Can you work these out from the drawing? Everything is in mm from the part's minimum corner. Give positions to 0.01 mm unless a question says otherwise; leave off trailing zeros. Write each loop counter-clockwise with the first axis right and the second up, starting at its lowest first coordinate (ties: lowest second). Pieces come first, ordered by that corner, then holes. Notation, with made-up numbers: (74, -20.5) - (97, -20.5) arc R29 cw to (97, 4.5) - close; hole circle Ø4 at (-2, 43.5). An arc over 180 degrees is marked (long way). Use a Markdown table: item, result.
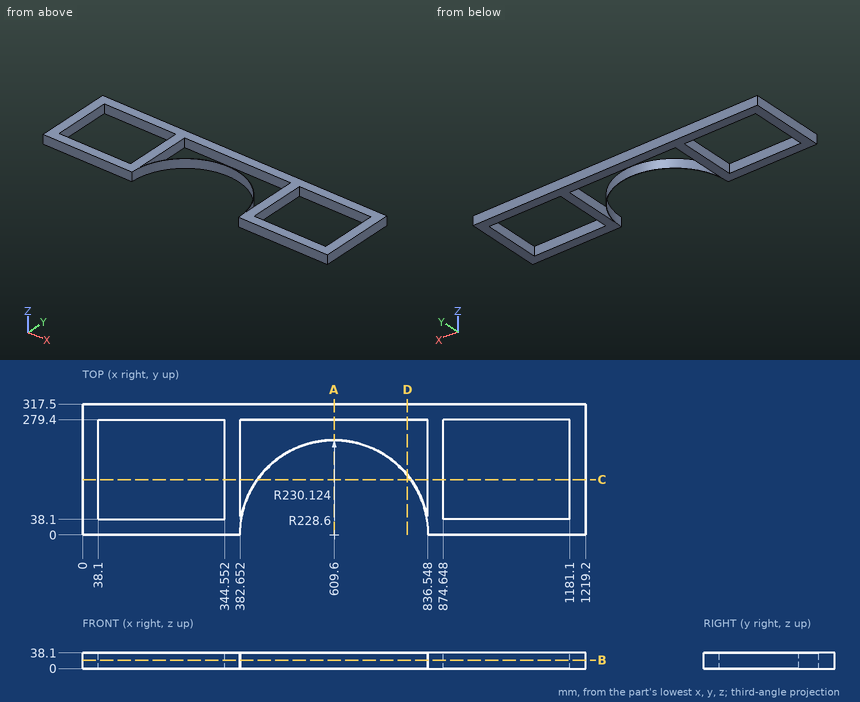
Item 1: If we section it at D-D, the plane x = 787.5: Write out the boundary of the cut face in (y, z) (3 decimals), plus the area to 3 significant figures.
Values:
| item | result |
|---|---|
| outline | (143.56, 0) - (145.975, 0) - (145.975, 38.1) - (143.56, 38.1) - close; (279.4, 0) - (317.5, 0) - (317.5, 38.1) - (279.4, 38.1) - close |
| area | 1,540 mm2 |
Item 2: If we section it at C-C, the plane y = 134: Write out the boundary of the cut face in (x, z).
Values:
| item | result |
|---|---|
| outline | (0, 0) - (38.1, 0) - (38.1, 38.1) - (0, 38.1) - close; (344.55, 0) - (382.65, 0) - (382.65, 38.1) - (344.55, 38.1) - close; (422.51, 0) - (424.39, 0) - (424.39, 38.1) - (422.51, 38.1) - close; (794.81, 0) - (796.69, 0) - (796.69, 38.1) - (794.81, 38.1) - close; (836.55, 0) - (874.65, 0) - (874.65, 38.1) - (836.55, 38.1) - close; (1181.1, 0) - (1219.2, 0) - (1219.2, 38.1) - (1181.1, 38.1) - close |
Item 3: If we section it at A-A, the plane x = 609.6: Write out the boundary of the cut face in (y, z).
Values:
| item | result |
|---|---|
| outline | (228.6, 0) - (230.12, 0) - (230.12, 38.1) - (228.6, 38.1) - close; (279.4, 0) - (317.5, 0) - (317.5, 38.1) - (279.4, 38.1) - close |
Item 4: Will this pin go through, and if not, where does the flat tip stop? pin 1 Ø19 at (x, z) = (533, 15) entering from -Y.
Values:
| item | result |
|---|---|
| pin 1 | stops at y = 211.77 |
Item 5: I need wall thicknesses on line 1 along Y through (x, z) = (118, 15.5); line 2 along X through (y, z) = (210, 11); line 3 along X through (y, z) = (160, 26). Which ranges of each line are inside material? Lowest first, please. Write a range as [from, to].
Values:
| item | result |
|---|---|
| line 1 | y = [0, 38.1], [279.4, 317.5] |
| line 2 | x = [0, 38.1], [344.55, 382.65], [515.49, 519.28], [699.92, 703.71], [836.55, 874.65], [1181.1, 1219.2] |
| line 3 | x = [0, 38.1], [344.55, 382.65], [444.2, 446.33], [772.87, 775], [836.55, 874.65], [1181.1, 1219.2] |
Item 6: If we section it at B-B, the plane z = 21: Write out the boundary of the cut face in (x, y).
Values:
| item | result |
|---|---|
| outline | (0, 0) - (381, 0) arc R228.6 cw to (838.2, 0) - (1219.2, 0) - (1219.2, 317.5) - (0, 317.5) - close; hole (38.1, 38.1) - (344.55, 38.1) - (344.55, 279.4) - (38.1, 279.4) - close; hole (382.65, 38.1) arc R230.12 cw to (836.55, 38.1) - (836.55, 279.4) - (382.65, 279.4) - close; hole (874.65, 38.1) - (1181.1, 38.1) - (1181.1, 279.4) - (874.65, 279.4) - close |
